Geometry check sheet. Reference: drawing and pictorial views, mm from the part's lowest x, y, z. Give positions to 0.01 mm unless a question says otherwise; leave off trailing zeros. Order: outer loops, then holes, each group sorted by start corner. A loop starts at its lowest first (then second) coordinate and runs counter-clockwise, first axis right, second up. Notation, with made-up numbers: (59, 4.5) - (70, 4.5) arc R14 ccw to (70, 8.5) - close; hole circle Ø3 at (5.5, -37). An arc over 180 degrees is marked (long way). Answer in a Markdown table with one row per item.
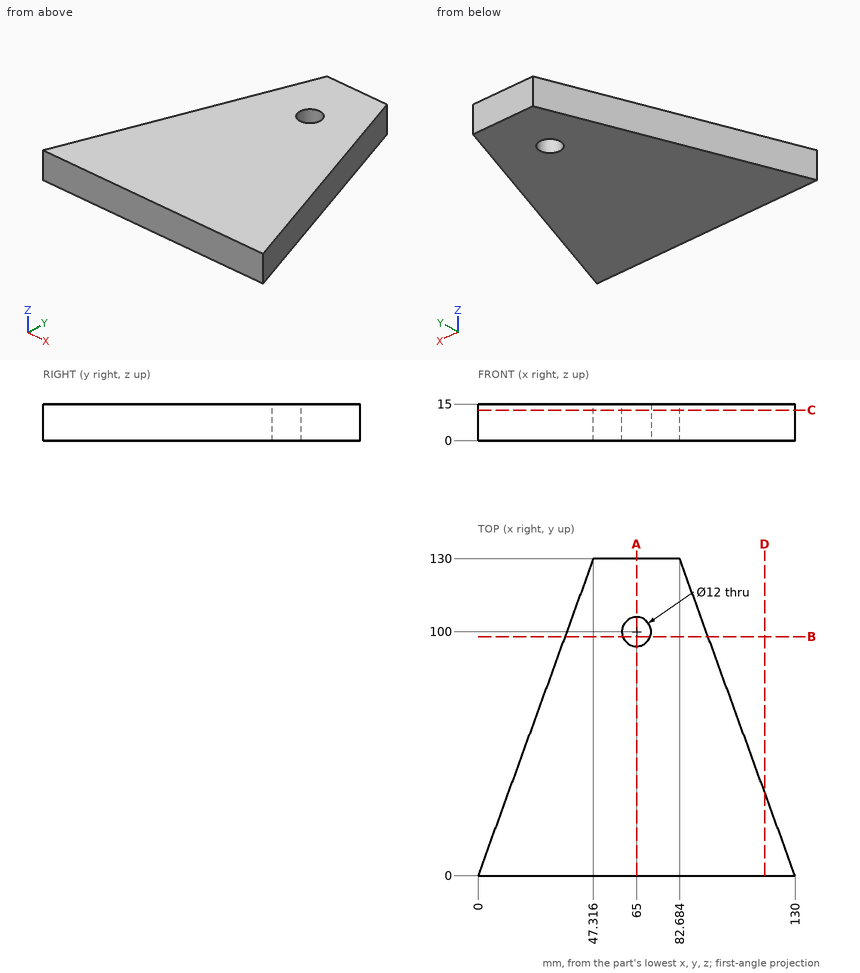
(1) Cross-section at D-D, the plane x = 117.5. Record the cut outline in (y, z).
Geometry says:
| item | result |
|---|---|
| outline | (0, 0) - (34.34, 0) - (34.34, 15) - (0, 15) - close |
(2) Thickness scan on L1, parallel to Y at x = 65, z = 7.5; L2, parallel to Y at x = 59.5, z = 6.25; L3, parallel to X at y = 94.5, z = 11.25 (1 decimal). Record the ranges inside material, lowest first.
Geometry says:
| item | result |
|---|---|
| L1 | 0 to 94, 106 to 130 |
| L2 | 0 to 97.6, 102.4 to 130 |
| L3 | 34.4 to 62.6, 67.4 to 95.6 |
(3) Cross-section at B-B, the plane y = 98. Record the cut outline in (x, z), then the cut area to 3 significant figures.
Geometry says:
| item | result |
|---|---|
| outline | (35.67, 0) - (59.34, 0) - (59.34, 15) - (35.67, 15) - close; (70.66, 0) - (94.33, 0) - (94.33, 15) - (70.66, 15) - close |
| area | 710 mm² |
(4) Gauge pin test, flat end, axial feed: P1, Ø1.5, axis at y = 56, z = 4.5, coming from the +X side. Record the tip position at first contact, or that the pin passes through.
Geometry says:
| item | result |
|---|---|
| P1 | x = 109.89 |
(5) Cross-section at C-C, the plane z = 12.5. Record the cut outline in (x, y), then the cut area to 3 significant figures.
Geometry says:
| item | result |
|---|---|
| outline | (0, 0) - (130, 0) - (82.68, 130) - (47.32, 130) - close; hole circle Ø12 at (65, 100) |
| area | 10,600 mm² |
(6) Cross-section at A-A, the plane x = 65. Record the cut outline in (y, z).
Geometry says:
| item | result |
|---|---|
| outline | (0, 0) - (94, 0) - (94, 15) - (0, 15) - close; (106, 0) - (130, 0) - (130, 15) - (106, 15) - close |
